Can you work these out from the model? Positions are in its coordinate system, mm. Coordinates: 2 decimals unless noted, no trailing zeros. Order: outer loops, then holes, each group sorted by start corner. A loop starts at its lowest first (then second) coordinate and runs counter-clockwise, first axis right, second up. Notation, with made-up numbers: M 72,-28.75 L 87,-28.75 A6 ccw 87,-22.75 Z; hole C -7,-32 d3. An arc over 180 degrees is marked long. Answer as a JSON object with one key per item and string values.
from build123d import *

# Parameters (mm, degrees)
SKETCH1_W           = 1706.88
SKETCH1_H           = 685.8
BOSS_EXTRUDE1_DEPTH = 7.62
SKETCH2_R           = 48.003123946
CUT_EXTRUDE1_DEPTH  = 7.62


with BuildPart() as part:
    # Sketch1 → Boss-Extrude1 (new body)
    with BuildSketch(Plane(origin=(0, 0, 0), x_dir=(1, 0, 0), z_dir=(0, 1, 0))):
        Rectangle(SKETCH1_W, SKETCH1_H)
    extrude(amount=BOSS_EXTRUDE1_DEPTH)

    # Sketch2 → Cut-Extrude1 (cut)
    with BuildSketch(Plane(origin=(0, 7.62, 0), x_dir=(1, 0, 0), z_dir=(0, 1, 0))):
        with Locations(Location((-775.698925032, 265.158925032, 0), (0, 0, 270))):
            Circle(SKETCH2_R)
        with BuildLine():
            Line((-780.493781084, 103.980830335), (-780.493781084, -103.980830335))
            ThreePointArc((-780.493781084, -103.980830335), (-799.17629755, -122.663346801), (-817.858814016, -103.980830335))
            Line((-817.858814016, -103.980830335), (-817.858814016, 103.980830335))
            ThreePointArc((-817.858814016, 103.980830335), (-799.17629755, 122.663346801), (-780.493781084, 103.980830335))
        make_face()
    extrude(amount=-CUT_EXTRUDE1_DEPTH, mode=Mode.SUBTRACT)


solid = part.part
Item 1: Please list where these lines run through material, in increasing order: line 1 (X direction, y = 1.5, z = -2); line 2 (Z direction, x = -748.5, y = 1.75); line 3 (X direction, y = 6.5, z = -280).
Answers follow:
{"line 1": "x = -853.44 to -817.86, -780.49 to 853.44", "line 2": "z = -342.9 to -304.71, -225.6 to 342.9", "line 3": "x = -853.44 to -821.35, -730.05 to 853.44"}
Item 2: If we mould it in two halves opening along Z, with no side actions, what happens to faces 1 (the cylindrical face through (-818.286, 3.863, -243.008)), 2 (the flat face through (-12, 7.62, -5))? For each: pulls with the +Z half, pulls with the -Z half, needs draft (parallel to the pull), parting line crosses it, or undercut.
Answers follow:
{"face 1": "undercut", "face 2": "needs draft"}
Item 3: I want a section at A-A, the plane z = -52.5. Write out the boundary of the cut face in (x, y).
Answers follow:
{"outline": "M -853.44,0 L -817.86,0 L -817.86,7.62 L -853.44,7.62 Z; M -780.49,0 L 853.44,0 L 853.44,7.62 L -780.49,7.62 Z"}
